Check sheet for the modelled part. Datum: model origin and axes. Units: mm. A direction names the side the tool comes from. Give positions to 0.01 mm unless a question says otherwise; leave off trailing zeros. Loops run counter-clockwise (first coordinate to the right, second up) from the corner with the lowest first, then second, coordinate; pieces in that order, holes last. Notation, with made-up numbers: (-26, 76) -> (17, 76) arc R21 cw to (17, 108) -> close; hole circle Ø7 at (36.5, -33.5). An arc over 180 degrees is marked (long way). Answer as CSV lines item,"result". Start each with the question number.
(1) Material ranges on line 1 (X direction, y = -3.25, z = 3.5); line 2 (X direction, y = -6, z = 0.25); line 3 (Z direction, x = 1.5, y = -6.25), recorded low to high. Write a range as from..to.
(2) Gauge pin test, flat ends, axial feed: pin 1 Ø4 at (y, z) = (-3, 7.5) entering from -X; pin 2 Ø1 at (x, y) = (6, -5.5) entering from -Z; pin 3 Ø3.5 at (x, z) = (-2, -2.5) entering from -Y. Record the tip position at first contact, or that the pin passes through.
(3) Section check B-B on x = 0. Enter the section's corners in (y, z).
(4) Access from +Z, -Z, +X, -X, +Y, -Y to the whole of each face (thin tool, end or side, straight path). Record for faces 4 (the face through (2, -7, -5)), 5 (the face through (0, -2.5, 0)).
(5) Section check A-A on y = -3.5. Enter the section's corners in (x, z).
(6) Section check D-D on y = -5.5. Enter the section's corners in (x, z).
(7) Release check for a two-part mould opening along Z. For faces 1 (the face through (3.234, -4.781, 3.813)), 2 (the face through (0, 0, 0)), 3 (the face through (6.78, -3.479, 10.635)) record: pulls with the +Z half, pulls with the -Z half, needs draft (parallel to the pull), parting line crosses it, or undercut.
(8) Section check C-C on z = 0. Enter the section's corners in (x, y), plus the area to 3 significant figures.
from build123d import *

# Parameters (mm, degrees)
F0_R     = 12.612488
F1_DEPTH = 7
F3_DEPTH = 4.5
F4_R     = 2


with BuildPart() as f1:
    # F0 (on Front) → F1 (new body)
    with BuildSketch(Plane.XZ):
        Circle(F0_R)
    extrude(amount=F1_DEPTH)

    # F2 (on face) → F3 (cut)
    with BuildSketch(Plane.XZ.offset(7)):
        Polygon((4.433325, -3.698508), (5.419665, 1.990118), (0.98634, 5.688626), (-4.433325, 3.698508), (-5.419665, -1.990118), (-0.98634, -5.688626), align=None)
    extrude(amount=-F3_DEPTH, mode=Mode.SUBTRACT)

    # F4
    f4_edges = [f1.edges().sort_by_distance(p)[0] for p in [
        (-12.612488, -7, 0),
        (-12.612488, 0, 0),
    ]]
    fillet(f4_edges, radius=F4_R)


solid = f1.part
Working result:
1,line 1,"x = -12.12..-4.47, 3.61..12.12"
1,line 2,"x = -12.34..-5.03, 5.12..12.34"
1,line 3,"z = -12.08..-4.78, 5.26..12.08"
2,pin 1,"stops at x = -11.35"
2,pin 2,"stops at z = -11.31"
2,pin 3,"stops at y = -2.5"
3,outline,"(-7, -10.61) arc R2 ccw to (-5, -12.61) -> (-2, -12.61) arc R2 ccw to (0, -10.61) -> (0, 10.61) arc R2 ccw to (-2, 12.61) -> (-5, 12.61) arc R2 ccw to (-7, 10.61) -> (-7, 5.33) -> (-2.5, 5.33) -> (-2.5, -5.33) -> (-7, -5.33) -> close"
4,face 4,"+Z, -Z, +X, -X, -Y"
4,face 5,"-Y"
5,outline,"circle Ø25.22 at (0, 0); hole (-5.42, -1.99) -> (-0.99, -5.69) -> (4.43, -3.7) -> (5.42, 1.99) -> (0.99, 5.69) -> (-4.43, 3.7) -> close"
6,outline,"circle Ø25.1 at (0, 0); hole (-5.42, -1.99) -> (-0.99, -5.69) -> (4.43, -3.7) -> (5.42, 1.99) -> (0.99, 5.69) -> (-4.43, 3.7) -> close"
7,face 1,"undercut"
7,face 2,"needs draft"
7,face 3,"parting line crosses it"
8,outline,"(-12.61, -5) arc R2 ccw to (-10.61, -7) -> (-5.07, -7) -> (-5.07, -2.5) -> (5.07, -2.5) -> (5.07, -7) -> (10.61, -7) arc R2 ccw to (12.61, -5) -> (12.61, -2) arc R2 ccw to (10.61, 0) -> (-10.61, 0) arc R2 ccw to (-12.61, -2) -> close"
8,area,"127 mm^2"
